from build123d import *

# Parameters (mm, degrees)
F1_DEPTH = 255.524
F2_R     = 127
F3_DEPTH = 254


with BuildPart() as f1:
    # F0 (on Top) → F1 (new body)
    with BuildSketch(Plane.XY):
        with BuildLine():
            ThreePointArc((395.4526, 0), (52.394599, 380.85148), (-333.5274, 43.50766))
            ThreePointArc((-333.5274, 43.50766), (-260.361114, -158.936751), (-60.56376, -239.04956))
            Line((-60.56376, -239.04956), (-31.5214, -239.04956))
            Line((-31.5214, -239.04956), (-31.5214, -303.3014))
            Line((-31.5214, -303.3014), (395.4526, -303.3014))
            Line((395.4526, -303.3014), (395.4526, 0))
        make_face()
    extrude(amount=F1_DEPTH)

    # F2 (on face) → F3 (join)
    with BuildSketch(Plane.XY.offset(255.524)):
        with Locations((-9.4234, -5.8674)):
            Circle(F2_R)
    extrude(amount=F3_DEPTH)

    # F6 (on face) → F9 (revolve)
    with BuildSketch(Plane.XZ.offset(5.8674)):
        with BuildLine():
            Line((121.1326, 509.524), (121.1326, 547.878))
            ThreePointArc((121.1326, 547.878), (113.693112, 565.838512), (95.7326, 573.278))
            Line((95.7326, 573.278), (-9.4234, 573.278))
            Line((-9.4234, 573.278), (-9.4234, 509.524))
            Line((-9.4234, 509.524), (121.1326, 509.524))
        make_face()
    revolve(axis=Axis((-9.4234, -5.8674, 525.207323), (0, 0, 1)))


solid = f1.part
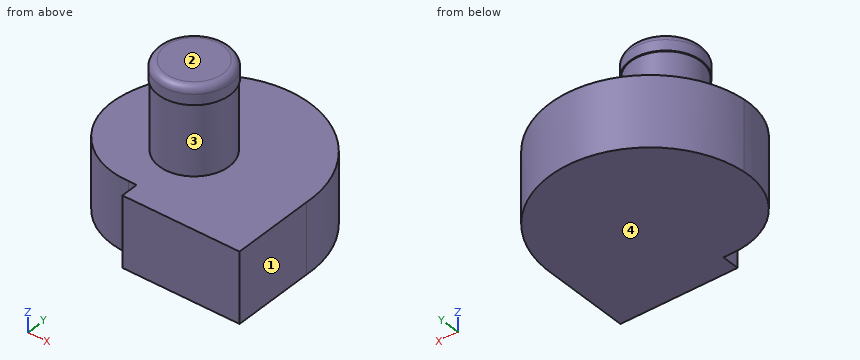
The listing builds one solid part. Answer for the finished solid, in the listing's coordinates (mm). Face numbers are marked on the shaded views. Give positions to 0.01 mm unless a question says otherwise; leave off trailing zeros. Order: outer loops, then holes, each group sorted by start corner. A loop starts at its lowest first (then second) coordinate and runs counter-clockwise, first axis right, second up. Notation, with made-up numbers: (20, 66.25) - (30, 66.25) arc R12 cw to (30, 87.25) - close; hole circle Ø5 at (74, 9). An arc over 180 degrees is marked (long way). One line per item, written item: value. Start each with the question number.
1) Find the intervals of material crossed by L1, parallel to Z at x = 297.5, y = -87; L2, parallel to Y at x = -6, z = 546; L3, parallel to X at y = -73.5, z = 45, in increasing order.
2) Given pin 1 Ø5 at (x, y) = (-98, 300.5) entering from +Z; pin 2 Ø1 at (y, z) = (123, 221.5) entering from -X; pin 3 Ø5 at (y, z) = (106, 422.5) entering from +X, each flat-ended and moving along its own axis, determine where each tip first touches the part or whether it passes through.
3) A cutting plane is placed at D-D on z = 390. Give the vertices of the cut face in (x, y).
4) A cutting plane is placed at C-C on y = 337. Give the vertices of the cut face in (x, z).
5) A cutting plane is placed at B-B on x = 160. Give the vertices of the cut face in (y, z).
6) The mould has two halves that part along Z. Classify the marked faces 1, 2, 3 and 4: released by +Z, released by -Z, zero draft, split by the parting line, or undercut.
7) A cutting plane is placed at A-A on z = 69. Give the vertices of the cut face in (x, y).
Answer sheet:
1. L1: z = 0 to 255.52
1. L2: y = -136.38 to 124.64
1. L3: x = -315.56 to 395.45
2. pin 1: stops at z = 255.52
2. pin 2: stops at x = -318.76
2. pin 3: stops at x = 55.13
3. outline: circle Ø254 at (-9.42, -5.87)
4. outline: (-144.06, 0) - (205.34, 0) - (205.34, 255.52) - (-144.06, 255.52) - close
5. outline: (-303.3, 0) - (357.82, 0) - (357.82, 255.52) - (-303.3, 255.52) - close
6. face 1: zero draft
6. face 2: released by +Z
6. face 3: undercut
6. face 4: released by -Z
7. outline: (-333.53, 43.51) arc R263.17 ccw to (-60.56, -239.05) - (-31.52, -239.05) - (-31.52, -303.3) - (395.45, -303.3) - (395.45, 0) arc R365.18 ccw to start
